Could you check a few things on this model? Use its own coordinates, in mm. Face numbers are marked on the shaded views. A direction names the side the tool comes from. Give positions to 0.01 mm unless a question says otherwise; leave off trailing zeros. Loops run counter-clockwise (first coordinate to the right, second up) from the corner with the lowest first, then second, coordinate; pieces in that order, holes last. Notation, with made-up numbers: M 36.25,-38 L 95.25,-38 A18 ccw 95.25,-19 Z; hole C 52.25,-30 d4. An arc over 180 degrees is marked long. Use a Markdown table: item, result. Add a question column.
1) Suppose I cut it at A-A on y = 286. List the corners of the cut face in (x, z) for me, and give its area (3 significant figures).
2) Suppose I cut it at B-B on x = 24. List the corners of the cut face in (y, z) for me, and give its area (3 significant figures).
3) If I drill on line 1 along Y through (x, z) = (22.5, 1.6); line 2 along X through (y, z) = (275.5, 1.6); line 3 along X through (y, z) = (273.5, 0.9), over which ranges is the centre line in solid material (lowest first)? Write a range as [from, to].
4) Suppose I cut it at C-C on y = 279.25. List the corners of the cut face in (x, z) for me.
5) We'd pull the mould along Y, two halves only. Please class the marked faces 1, 2 and 3: +Y half, -Y half, draft (parallel to the pull), parting line (faces both ways), or undercut.
6) Will these pins go through, and if not, where does the flat tip stop? pin 1 Ø0.5 at (x, z) = (27, 1) entering from +Y; pin 2 Ø2.5 at (x, y) = (21.17, 274.84) entering from -Z; pin 3 Ø5 at (x, y) = (21.17, 283.84) entering from -Z; pin 4 Ø0.9 at (x, z) = (16, 1) entering from -Y.
7) Which directions (+Z, -Z, +X, -X, +Y, -Y) give clear straight access to the entire face, cutting with the end or side of a thin tool? Please do the marked faces 4 and 5.
8) Suppose I cut it at D-D on z = 1.8. Count the separate pieces of the cut face and the enclosed holes in it, and give its area (3 significant figures).
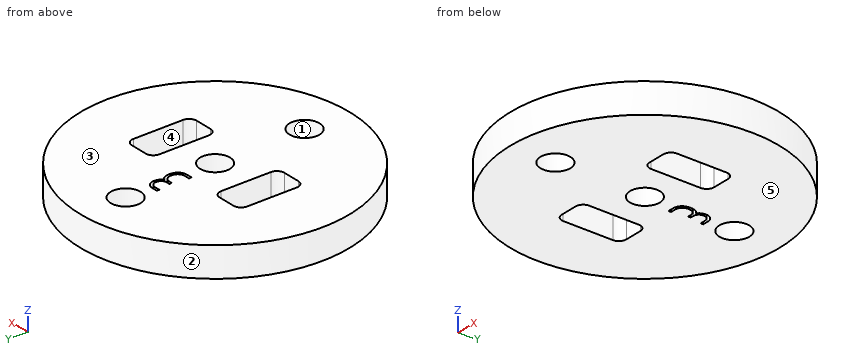
```python
from build123d import *

# Parameters (mm, degrees)
MODEL_R                 = 13.5
MODEL_R_2               = 1.5
SALIENTE_EXTRUIR1_DEPTH = 3


with BuildPart() as part:
    # Model → Saliente-Extruir1 (new body)
    with BuildSketch(Plane.XY):
        with Locations((21.167864369, 283.836969837)):
            Circle(MODEL_R)
        with Locations((21.167864369, 283.836969837)):
            Circle(MODEL_R_2, mode=Mode.SUBTRACT)
        with Locations((21.167864369, 292.836969837)):
            Circle(MODEL_R_2, mode=Mode.SUBTRACT)
        with Locations((21.167864369, 274.836969837)):
            Circle(MODEL_R_2, mode=Mode.SUBTRACT)
        with BuildLine():
            Line((27.542864369, 287.086969837), (25.792864369, 287.086969837))
            ThreePointArc((25.792864369, 287.086969837), (25.262534283, 286.867299923), (25.042864369, 286.336969837))
            Line((25.042864369, 286.336969837), (25.042864369, 281.336969837))
            ThreePointArc((25.042864369, 281.336969837), (25.262534283, 280.806639751), (25.792864369, 280.586969837))
            Line((25.792864369, 280.586969837), (27.542864369, 280.586969837))
            ThreePointArc((27.542864369, 280.586969837), (28.073194454, 280.806639751), (28.292864369, 281.336969837))
            Line((28.292864369, 281.336969837), (28.292864369, 286.336969837))
            ThreePointArc((28.292864369, 286.336969837), (28.073194454, 286.867299923), (27.542864369, 287.086969837))
        make_face(mode=Mode.SUBTRACT)
        with BuildLine():
            Line((14.792864369, 287.086969837), (16.542864369, 287.086969837))
            ThreePointArc((16.542864369, 287.086969837), (17.073194454, 286.867299923), (17.292864369, 286.336969837))
            Line((17.292864369, 286.336969837), (17.292864369, 281.336969837))
            ThreePointArc((17.292864369, 281.336969837), (17.073194454, 280.806639751), (16.542864369, 280.586969837))
            Line((16.542864369, 280.586969837), (14.792864369, 280.586969837))
            ThreePointArc((14.792864369, 280.586969837), (14.262534283, 280.806639751), (14.042864369, 281.336969837))
            Line((14.042864369, 281.336969837), (14.042864369, 286.336969837))
            ThreePointArc((14.042864369, 286.336969837), (14.262534283, 286.867299923), (14.792864369, 287.086969837))
        make_face(mode=Mode.SUBTRACT)
        with BuildLine():
            add(Edge.make_bspline(
                [(22.006993441, 287.753415048), (22.006172191, 287.716928587), (22.004568422, 287.645676392), (21.993135393, 287.541332376), (21.973516379, 287.442536499), (21.946685696, 287.348686497), (21.911477525, 287.260048048), (21.868040261, 287.176817115), (21.817632611, 287.098498345), (21.777884433, 287.05133063), (21.758042881, 287.027785384)],
                knots=[0, 0, 0, 0, 1.115577891, 2.178544379, 3.204804607, 4.192155228, 5.159249624, 6.11554861, 7.059316894, 8, 8, 8, 8], degree=3))
            add(Edge.make_bspline(
                [(21.758042881, 287.027785384), (21.73601152, 287.004605717), (21.692200482, 286.958511187), (21.617136147, 286.900352518), (21.537624651, 286.849328876), (21.451173506, 286.810051796), (21.359873554, 286.77752931), (21.262438119, 286.754808132), (21.159003088, 286.741929369), (21.088224879, 286.739885485), (21.05200277, 286.738839488)],
                knots=[0, 0, 0, 0, 0.974182212, 1.937235425, 2.888233128, 3.849890637, 4.826332808, 5.840933291, 6.895056104, 8, 8, 8, 8], degree=3))
            Line((21.05200277, 286.738839488), (20.497781687, 286.738839488))
            Line((20.497781687, 286.738839488), (20.497781687, 287.000033518))
            Line((20.497781687, 287.000033518), (21.033229449, 287.000033518))
            add(Edge.make_bspline(
                [(21.033229449, 287.000033518), (21.059653725, 287.000919571), (21.111355614, 287.002653229), (21.186916697, 287.013225583), (21.258244632, 287.031310058), (21.32576964, 287.056003306), (21.38961335, 287.087000578), (21.44975153, 287.124774673), (21.505586643, 287.169810236), (21.538837792, 287.204528413), (21.555617508, 287.222048443)],
                knots=[0, 0, 0, 0, 1.084178992, 2.121310725, 3.122997411, 4.097638005, 5.066122913, 6.029254004, 7.005491271, 8, 8, 8, 8], degree=3))
            add(Edge.make_bspline(
                [(21.555617508, 287.222048443), (21.570999544, 287.239956661), (21.601490979, 287.275455687), (21.639704379, 287.334170151), (21.672756978, 287.395771039), (21.699752927, 287.461072065), (21.72000496, 287.530104828), (21.73464822, 287.60219141), (21.743868039, 287.677813713), (21.745145683, 287.72944549), (21.745799411, 287.755863742)],
                knots=[0, 0, 0, 0, 0.975929627, 1.934561601, 2.891539334, 3.86584409, 4.852559224, 5.863826262, 6.906991381, 8, 8, 8, 8], degree=3))
            add(Edge.make_bspline(
                [(21.745799411, 287.755863742), (21.745351061, 287.782273605), (21.744471049, 287.834110399), (21.736907633, 287.91019579), (21.725020702, 287.982561288), (21.707666875, 288.051045489), (21.685633293, 288.115780826), (21.65874604, 288.177014822), (21.627095592, 288.234661565), (21.601696729, 288.269786427), (21.589082993, 288.287230346)],
                knots=[0, 0, 0, 0, 1.12360389, 2.205389034, 3.250364499, 4.241620612, 5.208228378, 6.156918895, 7.084678002, 8, 8, 8, 8], degree=3))
            add(Edge.make_bspline(
                [(21.589082993, 288.287230346), (21.574544546, 288.305301748), (21.545751158, 288.341092151), (21.495588333, 288.387456001), (21.441330602, 288.427404284), (21.381961231, 288.458984195), (21.318660617, 288.484833389), (21.250329767, 288.502552092), (21.177508361, 288.513371193), (21.127407132, 288.514421779), (21.101792881, 288.514958891)],
                knots=[0, 0, 0, 0, 0.994376019, 1.96936123, 2.922417962, 3.87868906, 4.848062798, 5.850838393, 6.901241263, 8, 8, 8, 8], degree=3))
            Line((21.101792881, 288.514958891), (20.753262098, 288.514958891))
            Line((20.753262098, 288.514958891), (20.753262098, 288.776152921))
            Line((20.753262098, 288.776152921), (21.10097665, 288.776152921))
            add(Edge.make_bspline(
                [(21.10097665, 288.776152921), (21.124978156, 288.776894886), (21.17221513, 288.778355134), (21.24067129, 288.791069119), (21.305723418, 288.810446517), (21.365901811, 288.839327455), (21.422358121, 288.875571718), (21.473959727, 288.920548215), (21.522716334, 288.97252323), (21.549889744, 289.0127191), (21.563779822, 289.033265794)],
                knots=[0, 0, 0, 0, 1.03852652, 2.043907225, 3.00545783, 3.969963621, 4.924268074, 5.901926174, 6.927539546, 8, 8, 8, 8], degree=3))
            add(Edge.make_bspline(
                [(21.563779822, 289.033265794), (21.580087317, 289.061494287), (21.613384605, 289.119132341), (21.626478423, 289.184420887), (21.633159486, 289.217734078)],
                knots=[0, 0, 0, 0, 0.9795089, 2, 2, 2, 2], degree=3))
            add(Edge.make_bspline(
                [(21.633159486, 289.217734078), (21.634295276, 289.22888413), (21.637116527, 289.256580356), (21.640596563, 289.306371742), (21.640310959, 289.372553775), (21.640961043, 289.422066995), (21.641321799, 289.449543779)],
                knots=[0, 0, 0, 0, 0.579519237, 1.439499501, 2.579080104, 4, 4, 4, 4], degree=3))
            add(Edge.make_bspline(
                [(21.641321799, 289.449543779), (21.640763207, 289.468644592), (21.63967018, 289.506020185), (21.628999757, 289.560636767), (21.614177359, 289.613425933), (21.590523941, 289.663107736), (21.562151141, 289.711395656), (21.525289358, 289.755836224), (21.484208987, 289.79980254), (21.452048145, 289.825137537), (21.435631501, 289.838069899)],
                knots=[0, 0, 0, 0, 1.002526936, 1.961698665, 2.916276685, 3.87598114, 4.844591571, 5.851696512, 6.903388936, 8, 8, 8, 8], degree=3))
            add(Edge.make_bspline(
                [(21.435631501, 289.838069899), (21.404492029, 289.859708178), (21.342724342, 289.902629473), (21.237809785, 289.945182436), (21.126620474, 289.972764119), (21.049727634, 289.975992976), (21.010374971, 289.977645458)],
                knots=[0, 0, 0, 0, 0.996493568, 1.9766264, 2.964466133, 4, 4, 4, 4], degree=3))
            Line((21.010374971, 289.977645458), (20.492068068, 289.977645458))
            Line((20.492068068, 289.977645458), (20.492068068, 290.238839488))
            Line((20.492068068, 290.238839488), (21.00384512, 290.238839488))
            add(Edge.make_bspline(
                [(21.00384512, 290.238839488), (21.050463483, 290.237830417), (21.140687736, 290.235877481), (21.270239549, 290.213980608), (21.388857916, 290.180083596), (21.496796805, 290.132553021), (21.593313097, 290.070012259), (21.677888732, 289.992796138), (21.753031972, 289.903301888), (21.79148527, 289.834697752), (21.811097919, 289.799707025)],
                knots=[0, 0, 0, 0, 1.150398076, 2.226457596, 3.234476189, 4.191097105, 5.1286688, 6.061241881, 7.011159392, 8, 8, 8, 8], degree=3))
            add(Edge.make_bspline(
                [(21.811097919, 289.799707025), (21.82509514, 289.770872206), (21.852143494, 289.715151544), (21.880625138, 289.629637364), (21.898956697, 289.546912649), (21.901352998, 289.492346985), (21.902515829, 289.465868406)],
                knots=[0, 0, 0, 0, 1.100306842, 2.126242689, 3.090738963, 4, 4, 4, 4], degree=3))
            add(Edge.make_bspline(
                [(21.902515829, 289.465868406), (21.901891131, 289.42775605), (21.900702296, 289.355226154), (21.891776806, 289.251582475), (21.8771786, 289.158564557), (21.861121354, 289.101169298), (21.853541949, 289.074077361)],
                knots=[0, 0, 0, 0, 1.154078597, 2.19627467, 3.148598438, 4, 4, 4, 4], degree=3))
            add(Edge.make_bspline(
                [(21.853541949, 289.074077361), (21.838843028, 289.036134419), (21.809139523, 288.959459511), (21.738416217, 288.854815662), (21.647160825, 288.759558716), (21.574488619, 288.706503935), (21.536844187, 288.679021391)],
                knots=[0, 0, 0, 0, 0.944683212, 1.909011131, 2.91686117, 4, 4, 4, 4], degree=3))
            add(Edge.make_bspline(
                [(21.536844187, 288.679021391), (21.556380181, 288.670189844), (21.595409564, 288.65254601), (21.650160169, 288.618471642), (21.70215206, 288.57948108), (21.749595699, 288.532763352), (21.794728064, 288.480789053), (21.835328975, 288.421709647), (21.872110759, 288.356686798), (21.893827459, 288.310775319), (21.904964523, 288.287230346)],
                knots=[0, 0, 0, 0, 0.931933608, 1.861834807, 2.799465617, 3.75391061, 4.752908839, 5.790647278, 6.866968556, 8, 8, 8, 8], degree=3))
            add(Edge.make_bspline(
                [(21.904964523, 288.287230346), (21.920920296, 288.247015558), (21.953322712, 288.165348797), (21.98404343, 288.034618703), (22.003330483, 287.896567742), (22.00575246, 287.801914037), (22.006993441, 287.753415048)],
                knots=[0, 0, 0, 0, 0.947814742, 1.924788424, 2.936695996, 4, 4, 4, 4], degree=3))
        make_face(mode=Mode.SUBTRACT)
    extrude(amount=SALIENTE_EXTRUIR1_DEPTH)


solid = part.part
```
Answer block:
| question | item | result |
|---|---|---|
| 1 | outline | M 7.84,0 L 14.04,0 L 14.04,3 L 7.84,3 Z; M 17.29,0 L 25.04,0 L 25.04,3 L 17.29,3 Z; M 28.29,0 L 34.49,0 L 34.49,3 L 28.29,3 Z |
| 1 | area | 60.5 mm^2 |
| 2 | outline | M 270.64,0 L 297.04,0 L 297.04,3 L 270.64,3 Z |
| 2 | area | 79.2 mm^2 |
| 3 | line 1 | y = [270.4, 274.15], [275.53, 283.15], [284.53, 292.15], [293.53, 297.27] |
| 3 | line 2 | x = [10.55, 19.82], [22.51, 31.79] |
| 3 | line 3 | x = [12.48, 20.49], [21.85, 29.85] |
| 4 | outline | M 8.47,0 L 33.86,0 L 33.86,3 L 8.47,3 Z |
| 5 | face 1 | undercut |
| 5 | face 2 | parting line |
| 5 | face 3 | draft |
| 6 | pin 1 | stops at y = 296.13 |
| 6 | pin 2 | passes through |
| 6 | pin 3 | stops at z = 0 |
| 6 | pin 4 | stops at y = 271.19 |
| 7 | face 4 | +Z, -Z |
| 7 | face 5 | -Z, +X, -X, +Y, -Y |
| 8 | separate pieces | 1 |
| 8 | enclosed holes | 6 |
| 8 | area | 508 mm^2 |
